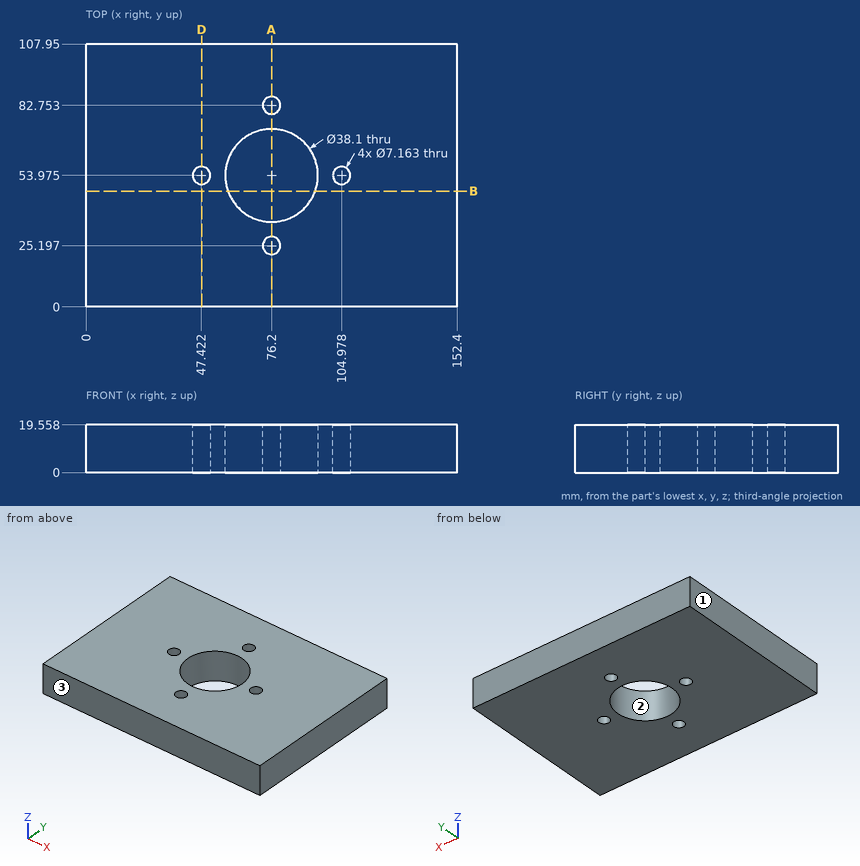
Study the drawing (mm; zero at the part's minimum x, y, z) and answer. Give positions to 0.01 mm unless a question says otherwise; leave off trailing zeros. Order: outer loops, then holes, each group sorted by start corner. A loop starts at its lowest first (then second) coordinate and runs counter-clockwise, first axis right, second up.
1) Find section B-B on y = 47.5. Write down the section's boundary in (x, z).
Reported:
outline: (0, 0) - (58.28, 0) - (58.28, 19.56) - (0, 19.56) - close; (94.12, 0) - (152.4, 0) - (152.4, 19.56) - (94.12, 19.56) - close
2) Find section D-D on x = 47.5. Write down the section's boundary in (y, z), then the cut area to 3 significant figures.
Reported:
outline: (0, 0) - (50.39, 0) - (50.39, 19.56) - (0, 19.56) - close; (57.56, 0) - (107.95, 0) - (107.95, 19.56) - (57.56, 19.56) - close
area: 1,970 mm2
3) Find section A-A on x = 76.2. Give the number of separate pieces and of enclosed holes in the cut face, then the cut area to 3 significant figures.
Reported:
separate pieces: 4
enclosed holes: 0
area: 1,090 mm2
4) Consider line 1 along Y through (x, z) = (76, 11.5); line 2 along X through (y, z) = (55.5, 18.25); line 3 along X through (y, z) = (54.5, 15.25) (1 decimal). Determine where each line is inside the solid, lowest interval first.
Reported:
line 1: y = 0 to 21.62, 28.77 to 34.93, 73.02 to 79.18, 86.33 to 107.95
line 2: x = 0 to 44.18, 50.66 to 57.21, 95.19 to 101.74, 108.22 to 152.4
line 3: x = 0 to 43.9, 51 to 57.2, 95.2 to 101.4, 108.5 to 152.4
5) Determine the mould class of the marked faces 1, 2 and 3 for opening direction X: pulls with the +X half, pulls with the -X half, needs draft (parallel to the pull), parting line crosses it, or undercut.
Reported:
face 1: pulls with the -X half
face 2: undercut
face 3: needs draft
